```python
from build123d import *

# Parameters (mm, degrees)
F1_DEPTH = 30
F2_R     = 1.5
F3_DEPTH = 21.001


with BuildPart() as f1:
    # F0 (on Front) → F1 (new body)
    with BuildSketch(Plane.XZ):
        Polygon((-8, 1), (0, 1), (8, 1), (9, 0), (17, 0), (17, 5), (15, 7), (15, 18), (6, 18), (3, 21), (0, 21), (-3, 21), (-6, 18), (-15, 18), (-15, 7), (-17, 5), (-17, 0), (-9, 0), align=None)
        with BuildLine():
            ThreePointArc((0, 15), (4, 11), (0, 7))
            ThreePointArc((0, 7), (-4, 11), (0, 15))
        make_face(mode=Mode.SUBTRACT)
    extrude(amount=F1_DEPTH)

    # F2 (on Top) → F3 (cut, through all)
    with BuildSketch(Plane.XY):
        with Locations((-12, -6.5)):
            Circle(F2_R)
        with Locations((-12, -23.5)):
            Circle(F2_R)
        with Locations((12, -23.5)):
            Circle(F2_R)
        with Locations((12, -6.5)):
            Circle(F2_R)
    extrude(amount=F3_DEPTH, mode=Mode.SUBTRACT)


solid = f1.part
```
Design review of the part built by this model. Coordinates are the model's own, in mm. A direction names the side the tool comes from. Give positions to 0.01 mm unless a question says otherwise; leave off trailing zeros. Write each loop counter-clockwise with the first axis right and the second up, starting at its lowest first coordinate (ties: lowest second). Pieces come first, ordered by that corner, then holes.
(1) Mouldability with a two-part tool opening along X and no side actions: class faces 5 (the face through (-8.5, -14.8, 0.5)), 6 (the face through (5, -15, 19)), 7 (the face through (-15, -15, 13)), 8 (the face through (13, -15, 0)) as +X half, -X half, draft (parallel to the pull), parting line (faces both ways), or undercut.
Checked values:
face 5: undercut
face 6: +X half
face 7: -X half
face 8: draft
(2) Add section D-D (z = 16). Give the boundary of the cut face in (x, y), and give its area (3 significant figures).
Checked values:
outline: (-15, -30) - (15, -30) - (15, 0) - (-15, 0) - close; hole circle Ø3 at (-12, -23.5); hole circle Ø3 at (-12, -6.5); hole circle Ø3 at (12, -23.5); hole circle Ø3 at (12, -6.5)
area: 872 mm2
(3) Add section C-C (x = 12). Give the boundary of the cut face in (y, z).
Checked values:
outline: (-30, 0) - (-25, 0) - (-25, 18) - (-30, 18) - close; (-22, 0) - (-8, 0) - (-8, 18) - (-22, 18) - close; (-5, 0) - (0, 0) - (0, 18) - (-5, 18) - close
(4) Add section A-A (z = 11). Give the boundary of the cut face in (x, y), and give its area (3 significant figures).
Checked values:
outline: (-15, -30) - (-4, -30) - (-4, 0) - (-15, 0) - close; (4, -30) - (15, -30) - (15, 0) - (4, 0) - close; hole circle Ø3 at (-12, -23.5); hole circle Ø3 at (-12, -6.5); hole circle Ø3 at (12, -23.5); hole circle Ø3 at (12, -6.5)
area: 632 mm2
(5) Clearance check with flat-ended pins moving along their axes: pin 1 Ø12 at (x, y) = (1.5, -13) entering from -Z; pin 2 Ø7 at (x, y) = (10.5, -17) entering from +Z; pin 3 Ø9 at (y, z) = (-8, 11) entering from +X. State where each tip first meets the part, or that it passes through.
Checked values:
pin 1: stops at z = 1
pin 2: stops at z = 18
pin 3: stops at x = 15.5
(6) Add section B-B (y = -23.5). Give the boundary of the cut face in (x, z).
Checked values:
outline: (-17, 0) - (-13.5, 0) - (-13.5, 18) - (-15, 18) - (-15, 7) - (-17, 5) - close; (-10.5, 0) - (-9, 0) - (-8, 1) - (8, 1) - (9, 0) - (10.5, 0) - (10.5, 18) - (6, 18) - (3, 21) - (-3, 21) - (-6, 18) - (-10.5, 18) - close; (13.5, 0) - (17, 0) - (17, 5) - (15, 7) - (15, 18) - (13.5, 18) - close; hole circle Ø8 at (0, 11)
(7) Wall thickness on line 1 along Y through (x, z) = (-12, 11.5); line 2 along X through (y, z) = (-23.5, 5.5); line 3 along Y through (x, z) = (-11, 16.75): over which ranges is each line inside the solid? List them lowest first.
Checked values:
line 1: y = -30 to -25, -22 to -8, -5 to 0
line 2: x = -16.5 to -13.5, -10.5 to 10.5, 13.5 to 16.5
line 3: y = -30 to -24.62, -22.38 to -7.62, -5.38 to 0
(8) Tool access review of faces 1 (the face through (11, -15, 18)), 2 (the face through (-13.2, -7.4, 8.9)), 3 (the face through (-10, -15, 18)), 4 (the face through (0, -15, 1)): name each direction out of +Z, -Z, +X, -X, +Y, -Y from which nothing blocks a thin tool from reaching the whole face with its end or side.
Checked values:
face 1: +Z, +X, +Y, -Y
face 2: +Z, -Z
face 3: +Z, -X, +Y, -Y
face 4: -Z, +Y, -Y
